Read the model definition and answer for the solid it produces. Units are mm, in the model's axes. Give positions to 0.01 mm unless a question says otherwise; leave off trailing zeros. Write each question's results on one line, items separated by ' | '. Start each with the question number.
Item 1: Section A-A on x = 27 is taken. State how many separate pieces and enclosed holes the cut face has, and give its area (3 significant figures).
Item 2: Find the intervals of material crossed by line 1 (Y direction, x = 18, z = 1.25); line 2 (Y direction, x = 16.5, z = 1.25); line 3 (X direction, y = 23, z = 3.5), in increasing order.
Item 3: Each of these flat-tipped pins is pushed along its axis until it touches: P1, Ø5, axis at x = 5.5, y = 128, coming from the +Z side; P2, Ø1.5, axis at x = 12, z = 4.5, coming from the +Y side; P3, Ø1.5, axis at y = 36, z = 1.5, coming from the -X side; P4, Ø3, axis at x = 25, z = 4, coming from the +Y side. Where does it stop, or does it pass through?
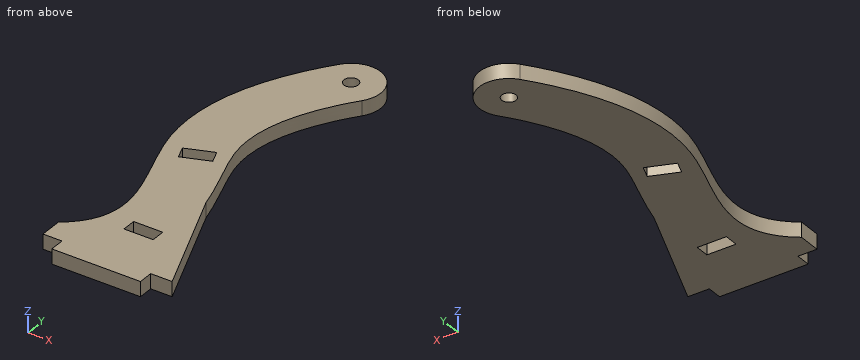
```python
from build123d import *

# Parameters (mm, degrees)
SKETCH1_R           = 3.0861
SKETCH1_W           = 12.5222
SKETCH1_H           = 5.9944
BOSS_EXTRUDE1_DEPTH = 6.35


with BuildPart() as part:
    # Sketch1 → Boss-Extrude1 (new body)
    with BuildSketch(Plane.XY):
        with BuildLine():
            Line((0, 0), (8.17063217, 0))
            Line((8.17063217, 0), (8.17063217, -6.35))
            Line((8.17063217, -6.35), (46.27063217, -6.35))
            Line((46.27063217, -6.35), (46.27063217, 0))
            Line((46.27063217, 0), (55.488574343, 0))
            Line((55.488574343, 0), (35.593928158, 49.97151257))
            add(Edge.make_bspline(
                [(35.593928158, 49.97151257), (35.340737153, 51.011091182), (34.289692424, 55.03884072), (31.957417171, 62.348344314), (29.449052089, 69.339178116), (27.57881277, 74.801296199), (26.423935243, 78.479850782), (25.55485091, 81.728738299), (24.788233703, 85.483659955), (24.284352637, 90.308612383), (24.428183006, 96.20335615), (25.327585112, 102.354497696), (27.029689584, 108.787993917), (29.577624998, 115.505437797), (32.431224266, 121.309144006), (35.158066015, 126.048842881), (37.424080544, 129.643418636), (39.497556945, 132.668231109), (41.261681964, 135.095684908), (42.186501173, 136.321547482), (42.651516027, 136.926910036)],
                knots=[0.250437186, 0.250437186, 0.250437186, 0.250437186, 0.266062186, 0.3125, 0.375, 0.40625, 0.4375, 0.46875, 0.5, 0.5625, 0.625, 0.6875, 0.75, 0.8125, 0.875, 0.90625, 0.9375, 0.96875, 0.984375, 1, 1, 1, 1], degree=3))
            ThreePointArc((42.651516027, 136.926910036), (40.316523303, 154.734992723), (22.508440616, 152.4))
            add(Edge.make_bspline(
                [(0, 9.589675689), (16.950704725, 21.543735705), (11.362052202, 46.597336486), (-7.636318626, 94.064001484), (3.941433469, 128.229221831), (22.508440616, 152.4)],
                knots=[0, 0, 0, 0, 0.312818519, 0.480279904, 1, 1, 1, 1], degree=3))
            Line((0, 9.589675689), (0, 0))
        make_face()
        with Locations((32.579978321, 144.663455018)):
            Circle(SKETCH1_R, mode=Mode.SUBTRACT)
        Polygon((8.17063217, 74.955854978), (10.310412852, 69.356375539), (22.007630495, 73.826341117), (19.867849812, 79.425820556), align=None, mode=Mode.SUBTRACT)
        with Locations((27.92484424, 22.035916142)):
            Rectangle(SKETCH1_W, SKETCH1_H, mode=Mode.SUBTRACT)
    extrude(amount=BOSS_EXTRUDE1_DEPTH)


solid = part.part
```
Findings:
1) separate pieces: 3 | enclosed holes: 0 | area: 792 mm2
2) line 1: -6.35 to 72.29, 78.71 to 146.22 | line 2: -6.35 to 71.72, 78.14 to 144 | line 3: 10.87 to 21.66, 34.19 to 46.33
3) P1: z = 6.35 | P2: y = 138.01 | P3: x = 12.22 | P4: y = 155.81
